Job drawing, mm, ordinate dimensions from the low corner. One solid piece. Coordinates: 2 decimals unless noted, no trailing zeros. Write each loop counter-clockwise with the first axis right and the second up, starting at its lowest first coordinate (ties: lowest second). Pieces come first, ordered by that corner, then holes. Notation, with made-up numbers: (42, -12) - (74, -12) arc R37 ccw to (74, 24) - close; hole circle Ø4 at (-5.75, -35.75). An arc over 180 degrees is marked (long way). Put each result on its own line as item: value. Start each with the question number.
1. Saw through at B-B, the plane y = 5.25. Give the number of separate pieces and of enclosed holes in the cut face, plus the area to 3 significant figures.
2. Drill centre lines: L1, parallel to X at y = 5.5, z = 18.5; L2, parallel to X at y = 3.25, z = 20.5; L3, parallel to Z at x = 49.5, y = 2. Where is each one in solid material? Low to high. Write a range as from..to.
3. Saw through at A-A, the plane z = 57.15. Write the cut outline in (x, y), plus the area to 3 significant figures.
4. Saw through at D-D, the plane z = 21. Write the cut outline in (x, y).
5. Saw through at C-C, the plane x = 86.5. Write the cut outline in (y, z).
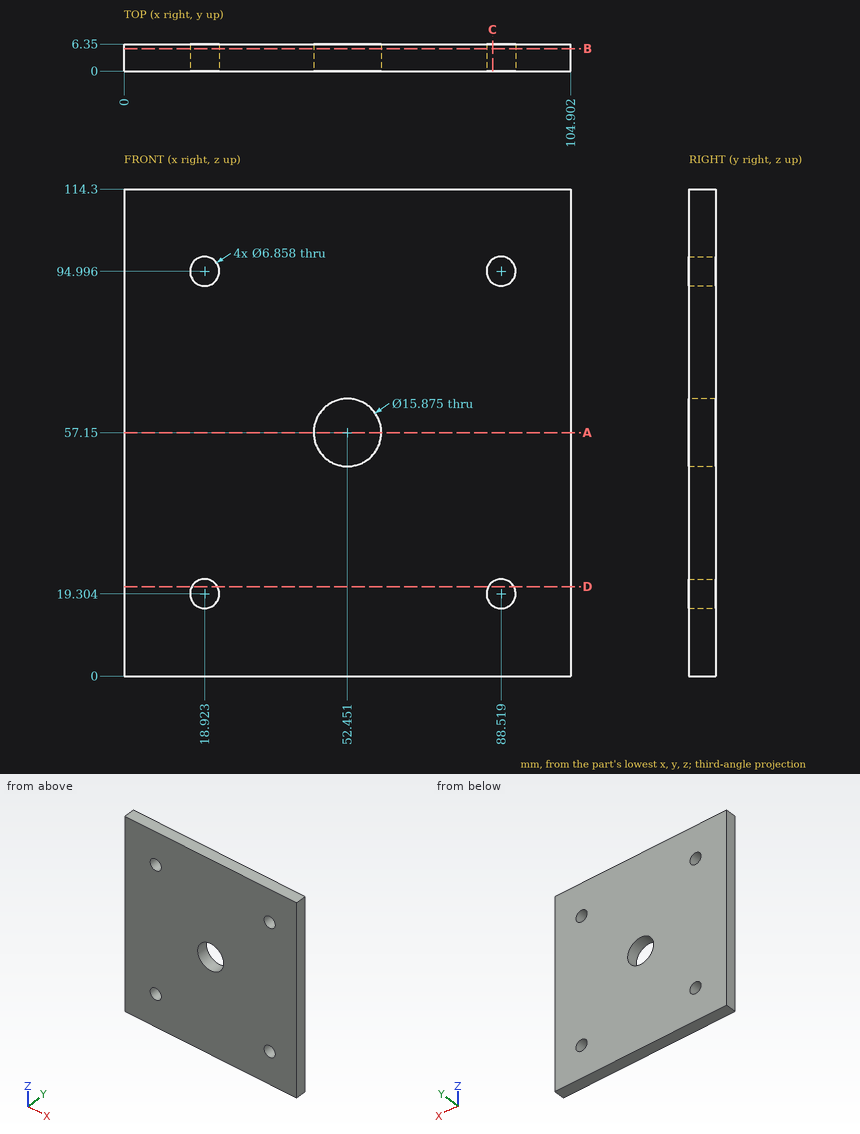
Final values:
1. separate pieces: 1
1. enclosed holes: 5
1. area: 11,600 mm²
2. L1: x = 0..15.59, 22.26..85.19, 91.85..104.9
2. L2: x = 0..15.71, 22.14..85.31, 91.73..104.9
2. L3: z = 0..49.78, 64.52..114.3
3. outline: (0, 0) - (44.51, 0) - (44.51, 6.35) - (0, 6.35) - close; (60.39, 0) - (104.9, 0) - (104.9, 6.35) - (60.39, 6.35) - close
3. area: 565 mm²
4. outline: (0, 0) - (15.94, 0) - (15.94, 6.35) - (0, 6.35) - close; (21.9, 0) - (85.54, 0) - (85.54, 6.35) - (21.9, 6.35) - close; (91.5, 0) - (104.9, 0) - (104.9, 6.35) - (91.5, 6.35) - close
5. outline: (0, 0) - (6.35, 0) - (6.35, 16.53) - (0, 16.53) - close; (0, 22.08) - (6.35, 22.08) - (6.35, 92.22) - (0, 92.22) - close; (0, 97.77) - (6.35, 97.77) - (6.35, 114.3) - (0, 114.3) - close
